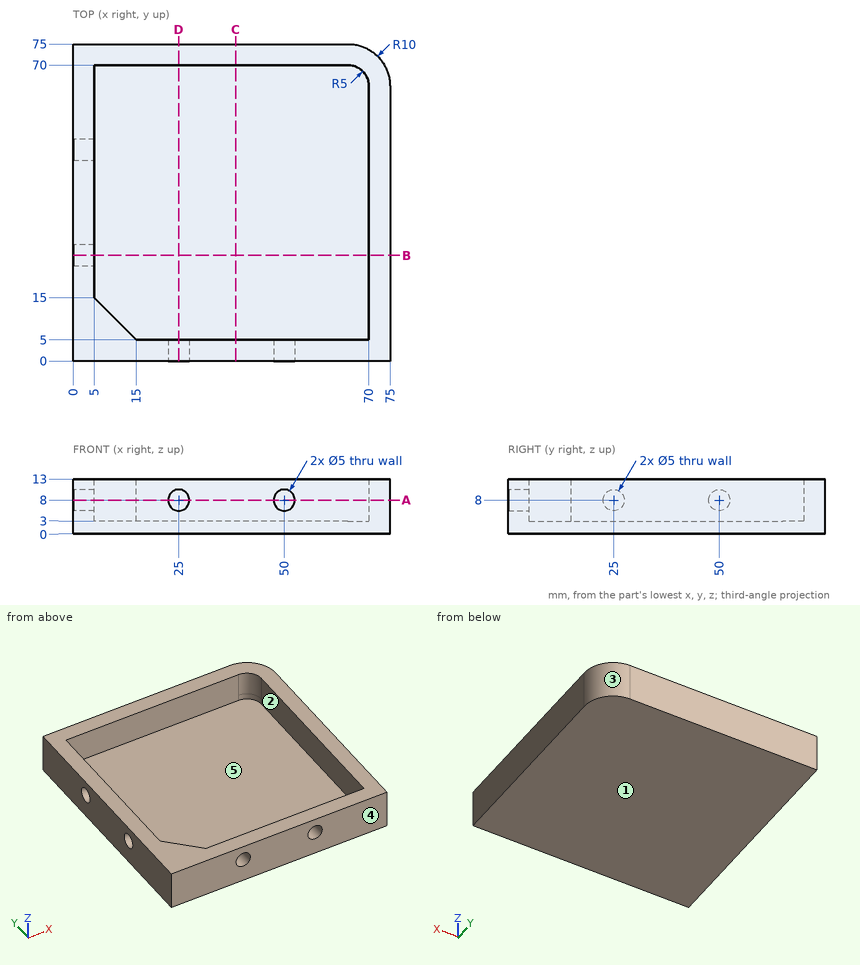
Answer from the drawing. Dimensions are ordinates in mm from the lowest x, y and z of the part. A direction names the side the tool comes from. Give positions to 0.01 mm unless a question says otherwise; leave off trailing zeros. Write each loop counter-clockwise with the first axis right and the second up, starting at its lowest first coordinate (ties: lowest second). Pieces come first, ordered by that corner, then holes. Notation, with made-up numbers: (58.5, 5.5) - (88.5, 5.5) arc R12 cw to (88.5, 26.5) - close; hole circle Ø1 at (54, 67.5). An arc over 180 degrees is marked (long way). Answer in a Markdown table with one row per item. Add a question column.
Item 1: Section B-B, the plane y = 25 is taken. Write down the section's boundary in (x, z).
Item 2: Determine the mould class of the marked faces 3, 4 and 5 for opening direction X: pulls with the +X half, pulls with the -X half, needs draft (parallel to the pull), parting line crosses it, or undercut.
Item 3: A tool of negligible diameter and unlimited length cuts with its end or side. For the marked faces 1 and 2, from which of +Z, -Z, +X, -X, +Y, -Y can it reach the whole face along a straight path? Write none if from no direction.
Item 4: Section C-C, the plane x = 38.5 is taken. Write down the section's boundary in (y, z), and give its area (3 significant figures).
Item 5: Section A-A, the plane z = 8 is taken. Write down the section's boundary in (x, y), and give its area (3 significant figures).
Item 6: Find the intervals of material crossed by L1, parallel to X at y = 1.5, z = 8; L2, parallel to Y at x = 14.5, z = 5.25; L3, parallel to X at y = 44, z = 12.5, in increasing order.
Recorded:
| question | item | result |
|---|---|---|
| 1 | outline | (0, 0) - (75, 0) - (75, 13) - (70, 13) - (70, 3) - (5, 3) - (5, 5.5) - (0, 5.5) - close; (0, 10.5) - (5, 10.5) - (5, 13) - (0, 13) - close |
| 2 | face 3 | pulls with the +X half |
| 2 | face 4 | needs draft |
| 2 | face 5 | undercut |
| 3 | face 1 | -Z, +X, -X, +Y, -Y |
| 3 | face 2 | +Z |
| 4 | outline | (0, 0) - (75, 0) - (75, 13) - (70, 13) - (70, 3) - (5, 3) - (5, 13) - (0, 13) - close |
| 4 | area | 325 mm2 |
| 5 | outline | (0, 0) - (22.5, 0) - (22.5, 5) - (15, 5) - (5, 15) - (5, 22.5) - (0, 22.5) - close; (0, 27.5) - (5, 27.5) - (5, 47.5) - (0, 47.5) - close; (0, 52.5) - (5, 52.5) - (5, 70) - (65, 70) arc R5 cw to (70, 65) - (70, 5) - (52.5, 5) - (52.5, 0) - (75, 0) - (75, 65) arc R10 ccw to (65, 75) - (0, 75) - close; (27.5, 0) - (47.5, 0) - (47.5, 5) - (27.5, 5) - close |
| 5 | area | 1,330 mm2 |
| 6 | L1 | x = 0 to 22.5, 27.5 to 47.5, 52.5 to 75 |
| 6 | L2 | y = 0 to 5.5, 70 to 75 |
| 6 | L3 | x = 0 to 5, 70 to 75 |
